Build history of the part. All positions in model axes, mm. Face numbers are marked on the shaded views. A direction names the side the tool comes from. Give positions to 0.01 mm unless a question says otherwise; leave off trailing zeros. Loops run counter-clockwise (first coordinate to the right, second up) from the corner with the lowest first, then second, coordinate; pieces in that order, holes last. Notation, with made-up numbers: M 66,52.25 L 96,52.25 A18 cw 96,63.25 Z; hole C 11,17 d2. An arc over 180 degrees is marked long. Put each result on its own line as item: value.
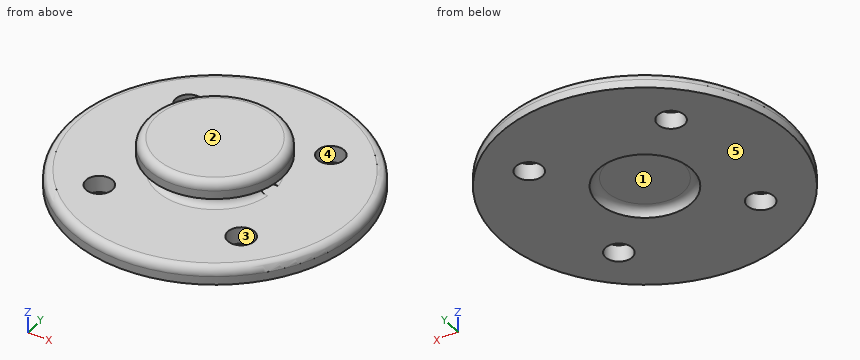
Autodesk Inventor part; units mm, degrees
ref_plane "YZ Plane" through (0, 0, 0) normal (1, 0, 0) x (0, 1, 0)
ref_plane "XZ Plane" through (0, 0, 0) normal (0, 1, 0) x (-1, 0, 0)
ref_plane "XY Plane" through (0, 0, 0) normal (0, 0, 1) x (1, 0, 0)
sketch "Sketch1" plane through (0, 0, 0) normal (0, 0, 1) x (1, 0, 0)
  circle A0 centre (0, 0) radius 8.7
  dimension "d0" = 17.4
extrude "Extrusion1" add sketch "Sketch1" along normal blind 1
sketch "Sketch2" plane through (0, 0, 1) normal (0, 0, 1) x (1, 0, 0)
  circle A0 centre (4.2426, 4.2426) radius 0.8
  circle A1 centre (-4.2426, 4.2426) radius 0.8
  circle A2 centre (-4.2426, -4.2426) radius 0.8
  circle A3 centre (4.2426, -4.2426) radius 0.8
  dimension "d9" = 1.6
  dimension "d10" = 1.6
  dimension "d11" = 1.6
  dimension "d12" = 1.6
extrude "Extrusion2" cut sketch "Sketch2" against normal up to next
sketch "Sketch3" plane through (0, 0, 0) normal (0, 0, -1) x (-1, 0, 0)
  circle A0 centre (0, 0) radius 2.8
  dimension "d15" = 5.6
extrude "Extrusion3" cut sketch "Sketch3" against normal blind 0.5
fillet "Fillet1" radius 0.5 1 edges at (2.8, 0, 0.5)
fillet "Fillet4" radius 0.5 1 edges at (-8.7, 0, 1)
sketch "Sketch7" plane through (0, 0, 1) normal (0, 0, 1) x (1, 0, 0)
  line L0 (-2.958, 0.5) -> (2.958, 0.5)
  line L1 (2.958, -0.5) -> (-2.958, -0.5)
  arc A0 (2.958, 0.5) -> (-2.958, 0.5) centre (0, 0) ccw
  arc A1 (-2.958, -0.5) -> (2.958, -0.5) centre (0, 0) ccw
  point P0 (0, 0)
extrude "Extrusion7" add sketch "Sketch7" along normal blind 1
sketch "Sketch8" plane through (0, 0, 2) normal (0, 0, 1) x (1, 0, 0)
  circle A0 centre (0, 0) radius 4
  dimension "d38" = 8
extrude "Extrusion8" add sketch "Sketch8" along normal blind 1
fillet "Fillet5" radius 0.5 4 edges at (0, -3, 2) (0, 3, 2) (0, 3, 1) (0, -3, 1)
fillet "Fillet6" radius 0.5 1 edges at (-4, 0, 3)
properties part number "pulley"
Q1. Tool access for the marked faces 1 and 2: list every direction of +Z, -Z, +X, -X, +Y, -Y with a clear straight run to the whole face (end or side of a thin tool).
Here are the results:
face 1: -Z
face 2: +Z, +X, -X, +Y, -Y
Q2. Mould opens along X. For the marked faces 3, 4 and 5 say: pulls with the +X half, pulls with the -X half, needs draft (parallel to the pull), parting line crosses it, or undercut.
Here are the results:
face 3: undercut
face 4: undercut
face 5: needs draft
Q3. Probe line 1 (Y direction, x = -4.25, z = 0.2); line 2 (Y direction, x = 0, z = 0.05); line 3 (Z direction, x = -1.5, y = 7.75). List the from-to ranges inside material, lowest first. Write a range as from..to.
Here are the results:
line 1: -7.59..-5.04, -3.44..3.44, 5.04..7.59
line 2: -8.7..-2.8, 2.8..8.7
line 3: 0..1
Q4. Drop flat-ended pins along their axis: pin 1 Ø5 at (x, y) = (0.5, 0.5) entering from -Z; pin 2 Ø2.5 at (x, y) = (4.24, -4.24) entering from +Z; pin 3 Ø1.5 at (y, z) = (-2, 2) entering from -X. Give the stop position or say it passes through.
Here are the results:
pin 1: z = 0
pin 2: z = 1
pin 3: x = -3.8
Q5. Slice it at C-C (z = 2.2). List the corners of the cut face in (x, y), and give its area (3 significant figures).
Here are the results:
outline: C 0,0 d8
area: 50.3 mm²
